```python
from build123d import *

# Parameters (mm, degrees)
SKETCH2_W           = 43
SKETCH2_H           = 37
SKETCH2_R           = 5
BOSS_EXTRUDE1_DEPTH = 12
SKETCH3_R           = 11
CUT_EXTRUDE1_DEPTH  = 7
SKETCH4_W           = 43
SKETCH4_H           = 34
BOSS_EXTRUDE2_DEPTH = 9
SKETCH5_R           = 1
CUT_EXTRUDE2_DEPTH  = 10


with BuildPart() as part:
    # Sketch2 → Boss-Extrude1 (new body)
    with BuildSketch(Plane.XY):
        with Locations((21.5, 18.5)):
            Rectangle(SKETCH2_W, SKETCH2_H)
        with Locations((21.5, 21)):
            Circle(SKETCH2_R, mode=Mode.SUBTRACT)
    extrude(amount=-BOSS_EXTRUDE1_DEPTH)

    # Sketch3 → Cut-Extrude1 (cut)
    with BuildSketch(Plane(origin=(0, 0, -12), x_dir=(-1, 0, 0), z_dir=(0, 0, -1))):
        with Locations((-21.5, 21)):
            Circle(SKETCH3_R)
    extrude(amount=-CUT_EXTRUDE1_DEPTH, mode=Mode.SUBTRACT)

    # Sketch4 → Boss-Extrude2 (add)
    with BuildSketch(Plane.XZ):
        with Locations((21.5, -17)):
            Rectangle(SKETCH4_W, SKETCH4_H)
    extrude(amount=-BOSS_EXTRUDE2_DEPTH)

    # Sketch5 → Cut-Extrude2 (cut)
    with BuildSketch(Plane.XY):
        with Locations((5.5, 5.5)):
            Circle(SKETCH5_R)
        with Locations((37.5, 5.5)):
            Circle(SKETCH5_R)
    extrude(amount=-CUT_EXTRUDE2_DEPTH, mode=Mode.SUBTRACT)


solid = part.part
```
Input: part model. Units: mm. Frame: model coordinates. A direction names the side the tool comes from. Coordinates: 2 decimals unless noted, no trailing zeros. Loops run counter-clockwise (first coordinate to the right, second up) from the corner with the lowest first, then second, coordinate; pieces in that order, holes last. Notation, with made-up numbers: M 51.25,-7 L 65.25,-7 A18 ccw 65.25,8 Z; hole C -37,2.5 d11. An arc over 180 degrees is marked long. One line per item, written item: value.
(1) Reachability of faces 5 (the flat face through (21, 37, -6)), 6 (the flat face through (16.8, 18.7, -5)), 7 (the flat face through (37, 6, -10)), 8 (the flat face through (21, 33, -12)) from +Z, -Z, +X, -X, +Y, -Y: full face, straight path, thin tool, end or side. Return the list, or none.
Filled in:
face 5: +Z, -Z, +X, -X, +Y
face 6: -Z
face 7: +Z
face 8: -Z, +X, -X, +Y
(2) Pin query (flat end, axial travel): pin 1 (1 mm diameter, centred on x = 27.5, y = 25, fed in from -Z); pin 2 (4 mm diameter, centred on x = 26, y = 29.5, fed in from -Z); pin 3 (1.8 mm diameter, centred on x = 37.5, y = 5.5, fed in from +Z); pin 4 (6.5 mm diameter, centred on x = 23, y = 20.5, fed in from -Z). Return the tip coordinate at first contact, or that it passes through.
Filled in:
pin 1: z = -5
pin 2: z = -12
pin 3: z = -10
pin 4: through
(3) Section A-A (y = 21). Output: boundary loops of the cut face in (x, z).
Filled in:
outline: M 0,-12 L 10.5,-12 L 10.5,-5 L 16.5,-5 L 16.5,0 L 0,0 Z; M 26.5,-5 L 32.5,-5 L 32.5,-12 L 43,-12 L 43,0 L 26.5,0 Z
(4) Section D-D (x = 8.5). Output: boundary loops of the cut face in (y, z), and give its area (3 significant figures).
Filled in:
outline: M 0,-34 L 9,-34 L 9,-12 L 37,-12 L 37,0 L 0,0 Z
area: 642 mm^2
(5) Pull-direction query (X, two-part tool) for faces 1 (the flat face through (43, 14, -10)), 2 (the cylindrical face through (11.339, 16.787, -8.549)), 3 (the flat face through (21, 0, -17)), 4 (the flat face through (0, 14, -10)); classes: +X half, -X half, draft (parallel to the pull), parting line (faces both ways), or undercut.
Filled in:
face 1: +X half
face 2: undercut
face 3: draft
face 4: -X half
(6) Section C-C (y = 5.5). Output: boundary loops of the cut face in (x, z), and give its area (3 significant figures).
Filled in:
outline: M 0,-34 L 43,-34 L 43,0 L 38.5,0 L 38.5,-10 L 36.5,-10 L 36.5,0 L 6.5,0 L 6.5,-10 L 4.5,-10 L 4.5,0 L 0,0 Z
area: 1,420 mm^2
(7) Section B-B (x = 21.5). Output: boundary loops of the cut face in (y, z), and give its area (3 significant figures).
Filled in:
outline: M 0,-34 L 9,-34 L 9,-12 L 10,-12 L 10,-5 L 16,-5 L 16,0 L 0,0 Z; M 26,-5 L 32,-5 L 32,-12 L 37,-12 L 37,0 L 26,0 Z
area: 438 mm^2
(8) Line query: line 1 along Y through (x, z) = (37.5, -5.25); line 2 along Y through (x, z) = (8.5, -14); line 3 along Y through (x, z) = (21.5, -1.2). Output: solid intervals per line, ascending. Write a range as from..to.
Filled in:
line 1: 0..4.5, 6.5..37
line 2: 0..9
line 3: 0..16, 26..37
